Can you work these out from the model? Positions are in its coordinate system, mm. A direction names the side the tool comes from. Coordinates: 2 decimals unless noted, no trailing zeros. Write each loop counter-clockwise with the first axis right and the second up, starting at its lowest first coordinate (ties: lowest second). Pieces come first, ordered by that corner, then holes. Notation, with made-up numbers: (23, 86.5) - (32, 86.5) arc R17 ccw to (32, 112.5) - close; hole circle Ø10 at (18.5, -5.5). An arc over 180 degrees is marked (long way). Write each question's results on one line, items separated by ' | '. Start each with the question number.
```python
from build123d import *

# Parameters (mm, degrees)
CHAMFER1_SIZE = 0.508


with BuildPart() as part:
    # Sketch1 → Revolve1 (revolve)
    with BuildSketch(Plane.XY, mode=Mode.PRIVATE) as revolve1_sk:
        Polygon((-38.510306737, 2.281775494), (-37.748306737, 2.281775494), (-37.748306737, -1.686974506), (-33.430306737, -1.686974506), (-27.080306737, -1.686974506), (-27.080306737, -3.433224506), (-31.144306737, -3.433224506), (-31.144306737, -4.068224506), (-38.510306737, -4.068224506), align=None)
    revolve(revolve1_sk.sketch.rotate(Axis((-27.588306737, -7.243224506, 0), (1, 0, 0)), 90), axis=Axis((-27.588306737, -7.243224506, 0), (1, 0, 0)))

    # Chamfer1
    chamfer1_edges = [part.edges().sort_by_distance(p)[0] for p in [
        (-38.510306737, -7.243224506, -3.175),
        (-38.510306737, -7.243224506, -9.525),
        (-27.080306737, -7.243224506, -3.81),
    ]]
    chamfer(chamfer1_edges, length=CHAMFER1_SIZE)


solid = part.part
```
Q1. For faces 5 (the face through (-37.748, -3, 4)), 6 (the face through (-34.62, -10.39, -0.41)), which set-ups out of +Z, -Z, +X, -X, +Y, -Y let a thin tool reach every point of the face, with its end or its side?
Q2. I'm going to push flat-ended pins straight in: pin 1 Ø4 at (x, z) = (-32, 5.5) entering from +Y; pin 2 Ø6 at (x, y) = (-34, -0.5) entering from -Z; pin 3 Ø2 at (x, z) = (-34, 5.5) entering from -Y. Where does each tip first touch, or does it pass through?
Q3. If we section it at B-B (x = -28): Please give me the cut outline in (y, z), then the cut area to 3 significant figures.
Q4. If we section it at A-A (z = 0): Please give me the cut outline in (x, y).
Q5. Thinking about a two-plate mould opening in Y: for faces 1 (the face through (-31.144, -10, -2)), 2 (the face through (-32.49, -1.82, -1.2)), 3 (the face through (-27.08, -2.7, 0)), 4 (the face through (-29.391, -10.456, 2.048)), which applies, pulls with the +Y half, pulls with the -Y half, needs draft (parallel to the pull), parting line crosses it, or undercut?
Q6. I need wall thicknesses on line 1 along Y through (x, z) = (-28.8, 0); line 2 along Y through (x, z) = (-32.5, 0); line 3 along X through (y, z) = (-0.75, 3.25). Which ranges of each line are inside material? Lowest first, please. Write a range as from..to.
Answer list:
1) face 5: +X | face 6: +X, -X
2) pin 1: stops at y = -2.93 | pin 2: stops at z = -4.11 | pin 3: stops at y = -10.5
3) outline: circle Ø11.11 at (-7.24, 0); hole circle Ø7.62 at (-7.24, 0) | area: 51.4 mm2
4) outline: (-38.51, -16.26) - (-38, -16.77) - (-37.75, -16.77) - (-37.75, -12.8) - (-27.08, -12.8) - (-27.08, -11.56) - (-27.59, -11.05) - (-31.14, -11.05) - (-31.14, -10.42) - (-38, -10.42) - (-38.51, -10.93) - close; (-38.51, -3.56) - (-38, -4.07) - (-31.14, -4.07) - (-31.14, -3.43) - (-27.59, -3.43) - (-27.08, -2.93) - (-27.08, -1.69) - (-37.75, -1.69) - (-37.75, 2.28) - (-38, 2.28) - (-38.51, 1.77) - close
5) face 1: undercut | face 2: parting line crosses it | face 3: needs draft | face 4: undercut
6) line 1: y = -12.8..-11.05, -3.43..-1.69 | line 2: y = -12.8..-10.42, -4.07..-1.69 | line 3: x = -38.51..-37.75
